Verification items for the finished model (mm, model axes). Round coordinates to 2 decimals unless told otherwise and drop trailing zeros. Write each loop counter-clockwise with the first axis right and the second up, starting at its lowest first coordinate (ties: lowest second). Pieces come first, ordered by that corner, then holes.
Autodesk Inventor part; units mm, degrees
ref_plane "YZ Plane" through (0, 0, 0) normal (1, 0, 0) x (0, 1, 0)
ref_plane "XZ Plane" through (0, 0, 0) normal (0, 1, 0) x (-1, 0, 0)
ref_plane "XY Plane" through (0, 0, 0) normal (0, 0, 1) x (1, 0, 0)
sketch "Sketch1" plane through (0, 0, 0) normal (0, 0, 1) x (1, 0, 0)
  circle A0 centre (0, 0) radius 20.775
  circle A1 centre (0, 0) radius 19.6781
  dimension "d9" = 1.0969
  dimension "d10" = 41.55
extrude "Extrusion1" add sketch "Sketch1" along normal mid plane 17.8
chamfer "Chamfer1" distance 1 angle 45 1 edges at (-19.6781, 0, 8.9)
sketch "Sketch2" plane through (0, 0, -8.9) normal (0, 0, -1) x (-1, 0, 0)
  circle A0 centre (0, 0) radius 21.8479
extrude "Extrusion2" cut sketch "Sketch2" against normal blind 1.5
sketch "Sketch3" plane through (0, 0, 0) normal (1, 0, 0) x (0, 1, 0)
  circle A0 centre (0, -5.7538) radius 0.6488
  point P0 (0, 0)
extrude "Extrusion3" cut sketch "Sketch3" against normal mid plane 100
properties part number "_3DPrint"
Q1. Material ranges on line 1 along Y through (x, z) = (-0.5, 7.75); line 2 along X through (y, z) = (0, -1) (3 decimals); line 3 along X through (y, z) = (2, 1.25), recorded low to high.
Recorded:
line 1: y = -20.77 to -19.67, 19.67 to 20.77
line 2: x = -20.775 to -19.678, 19.678 to 20.775
line 3: x = -20.68 to -19.58, 19.58 to 20.68
Q2. Sectioned sample at A-A (y = 0). Enter the section's corners in (x, z) (3 decimals).
Recorded:
outline: (-20.775, -7.4) - (-19.678, -7.4) - (-19.678, -6.403) - (-20.775, -6.403) - close; (-20.775, -5.105) - (-19.678, -5.105) - (-19.678, 7.9) - (-20.678, 8.9) - (-20.775, 8.9) - close; (19.678, -7.4) - (20.775, -7.4) - (20.775, -6.403) - (19.678, -6.403) - close; (19.678, -5.105) - (20.775, -5.105) - (20.775, 8.9) - (20.678, 8.9) - (19.678, 7.9) - close
Q3. Release check for a two-part mould opening along Y. For faces 1 (the cylindrical face through (11.169, -17.518, 0.636)), 2 (the flat face through (-7.6, -18.4, -7.4)), 3 (the cylindrical face through (18.178, 7.537, 0.143)) record: released by +Y, released by -Y, zero draft, split by the parting line, or undercut.
Recorded:
face 1: split by the parting line
face 2: zero draft
face 3: undercut
Q4. Depth check by flat-ended pin: P1, Ø5, axis at y = -15, z = -1.5, coming from the +X side; P2, Ø4, axis at y = 15, z = 3.5, coming from the -X side; P3, Ø4, axis at x = -12, z = -3, coming from the +Y side. Enter the tip coordinate at first touch or a pass-through.
Recorded:
P1: stops at x = 16.59
P2: stops at x = -16.2
P3: stops at y = 18.21
Q5. Sectioned sample at C-C (z = 6). Enter the section's corners in (x, y) (3 decimals), plus the area to 3 significant figures.
Recorded:
outline: circle Ø41.55 at (0, 0); hole circle Ø39.356 at (0, 0)
area: 139 mm2
Q6. Sectioned sample at B-B (x = 0). Enter the section's corners in (y, z) (3 decimals).
Recorded:
outline: (-20.775, -7.4) - (-19.678, -7.4) - (-19.678, 7.9) - (-20.678, 8.9) - (-20.775, 8.9) - close; (19.678, -7.4) - (20.775, -7.4) - (20.775, 8.9) - (20.678, 8.9) - (19.678, 7.9) - close
